Work out the finished part from the listing and answer in its coordinate system (mm). Face numbers are marked on the shaded views. A direction names the side the tool comes from. Round coordinates to 2 decimals unless told otherwise and drop trailing zeros. Loops run counter-clockwise (first coordinate to the right, second up) from the corner with the lowest first, then second, coordinate; pieces in that order, holes last. Notation, with made-up numbers: (-21, -1.5) - (30, -1.5) arc R28 cw to (30, 37.5) - close; hole circle Ø4 at (-20.5, 11.5). An arc over 180 degrees is marked (long way). Answer as CSV lines item,"result". Start each with the question number.
Q1. For the marked faces 1, 2 and 3, determine the directions among +Z, -Z, +X, -X, +Y, -Y from which every point of the face is accessible in a straight line to the end or side of a thin tool.
Q2. Section A-A on z = -5 is taken. Write down the section's boundary in (x, y), then the cut area to 3 significant figures.
Q3. Section C-C on y = 0.5 is taken. Write down the section's boundary in (x, z) (3 decimals), then the cut area to 3 significant figures.
Q4. Straight lines are drawn through the part: L1, parallel to X at y = 1.5, z = 17.78 (3 decimals); L2, parallel to Z at x = -20.32, y = -1.75; L3, parallel to X at y = 0.25, z = 4.5. For each, find the intervals that lie inside material, in ascending order. Write a range as [from, to].
Q5. Each of these flat-tipped pins is pushed along its axis until it touches: pin 1 Ø3 at (x, z) = (-17, -1) entering from -Y; pin 2 Ø1.4 at (x, z) = (-20.32, -17.78) entering from -Y; pin 3 Ø3 at (x, y) = (-2, 2) entering from -Z; pin 4 Ø3.5 at (y, z) = (-1, 18.5) entering from +X. Where does it stop, or does it pass through?
Q6. Section B-B on x = 0 is taken. Write down the section's boundary in (y, z).
Q7. The mould has two halves that part along X. Classify the marked faces 4, 5 and 6: +X half, -X half, draft (parallel to the pull), parting line (faces both ways), or undercut.
Q8. Section D-D on y = -6 is taken. Write down the section's boundary in (x, z), then the cut area to 3 significant figures.
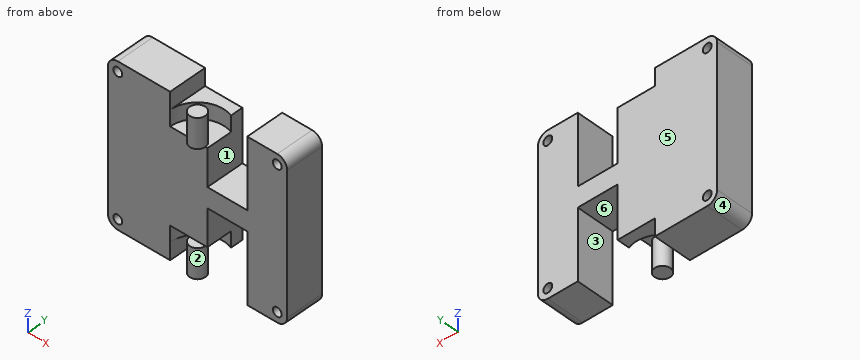
```python
from build123d import *

# Parameters (mm, degrees)
SKETCH1_W             = 45.72
SKETCH1_H             = 40.64
BODY_DEPTH            = 4.826
CORNER_FILLET_R       = 2.54
F_4_40_TAPPED_HOLE1_D = 2.2606
SKETCH4_W             = 13.97
SKETCH4_H             = 9.652
WHEEL_CUTOUT_DEPTH    = 8.382
SKETCH5_R             = 2
WHEEL_SHAFT_DEPTH     = 7.5
SKETCH9_W             = 10.16
SKETCH9_H             = 9.652
CUT_EXTRUDE2_DEPTH    = 17.78
BOSS_EXTRUDE2_DEPTH   = 4


with BuildPart() as part:
    # Sketch1 → Body (new body, symmetric)
    with BuildSketch(Plane(origin=(0, 0, 0), x_dir=(1, 0, 0), z_dir=(0, 1, 0))):
        Rectangle(SKETCH1_W, SKETCH1_H)
    extrude(amount=BODY_DEPTH, both=True)

    # Corner Fillet
    corner_fillet_edges = [part.edges().sort_by_distance(p)[0] for p in [
        (22.86, 0, 20.32),
        (-22.86, 0, 20.32),
        (-22.86, 0, -20.32),
        (22.86, 0, -20.32),
    ]]
    fillet(corner_fillet_edges, radius=CORNER_FILLET_R)

    # #4-40 Tapped Hole1 (through all)
    with Locations(Plane(origin=(0, 4.826, 0), x_dir=(1, 0, 0), z_dir=(0, 1, 0))):
        with Locations((20.32, 17.78), (-20.32, -17.78), (-20.32, 17.78), (20.32, -17.78)):
            Hole(F_4_40_TAPPED_HOLE1_D / 2)

    # Sketch4 → Wheel Cutout (cut)
    with BuildSketch(Plane(origin=(0, 0, -20.32), x_dir=(-1, 0, 0), z_dir=(0, 0, -1))):
        Rectangle(SKETCH4_W, SKETCH4_H)
    wheel_cutout = extrude(amount=-WHEEL_CUTOUT_DEPTH, mode=Mode.SUBTRACT)

    # Sketch5 → Wheel Shaft (add)
    with BuildSketch(Plane(origin=(0, 0, -11.938), x_dir=(-1, 0, 0), z_dir=(0, 0, -1))):
        with Locations((0, -4.826)):
            Circle(SKETCH5_R)
    wheel_shaft = extrude(amount=WHEEL_SHAFT_DEPTH)

    # Sketch9 → Cut-Extrude2 (cut)
    with BuildSketch(Plane(origin=(0, 0, -20.32), x_dir=(-1, 0, 0), z_dir=(0, 0, -1))):
        with Locations((-7.603288762, 0)):
            Rectangle(SKETCH9_W, SKETCH9_H)
    cut_extrude2 = extrude(amount=-CUT_EXTRUDE2_DEPTH, mode=Mode.SUBTRACT)

    # Sketch10 → Boss-Extrude2 (add)
    with BuildSketch(Plane(origin=(0, 0, -11.938), x_dir=(-1, 0, 0), z_dir=(0, 0, -1))):
        with BuildLine():
            Line((6.985, 4.826), (-2.523288762, 4.826))
            Line((-2.523288762, 4.826), (-2.523288762, 1.687312431))
            ThreePointArc((-2.523288762, 1.687312431), (3.947470899, 0.936612125), (6.985, -4.826))
            Line((6.985, -4.826), (6.985, 4.826))
        make_face()
    boss_extrude2 = extrude(amount=BOSS_EXTRUDE2_DEPTH)

    # Mirror3: Wheel Cutout, Wheel Shaft, Cut-Extrude2, Boss-Extrude2 across plane
    add(wheel_cutout.mirror(Plane.XY), mode=Mode.SUBTRACT)
    add(wheel_shaft.mirror(Plane.XY))
    add(cut_extrude2.mirror(Plane.XY), mode=Mode.SUBTRACT)
    add(boss_extrude2.mirror(Plane.XY))


solid = part.part
```
Findings:
1,face 1,"+Z, +Y, -Y"
1,face 2,"-Z"
1,face 3,"-Z, +Y, -Y"
2,outline,"(-22.86, -4.83) - (2.52, -4.83) - (2.52, 4.83) - (-22.86, 4.83) - close; (12.68, -4.83) - (22.86, -4.83) - (22.86, 4.83) - (12.68, 4.83) - close"
2,area,"343 mm^2"
3,outline,"(-22.86, -17.78) arc R2.54 ccw to (-20.32, -20.32) - (-6.985, -20.32) - (-6.985, -15.938) - (-4.519, -15.938) - (-4.519, -11.938) - (2.523, -11.938) - (2.523, -2.54) - (12.683, -2.54) - (12.683, -20.32) - (20.32, -20.32) arc R2.54 ccw to (22.86, -17.78) - (22.86, 17.78) arc R2.54 ccw to (20.32, 20.32) - (12.683, 20.32) - (12.683, 2.54) - (2.523, 2.54) - (2.523, 11.938) - (-4.519, 11.938) - (-4.519, 15.938) - (-6.985, 15.938) - (-6.985, 20.32) - (-20.32, 20.32) arc R2.54 ccw to (-22.86, 17.78) - close; hole circle Ø2.261 at (-20.32, -17.78); hole circle Ø2.261 at (-20.32, 17.78); hole circle Ø2.261 at (20.32, -17.78); hole circle Ø2.261 at (20.32, 17.78)"
3,area,"1,340 mm^2"
4,L1,"x = [-22.86, -21.45], [-19.19, -6.985], [12.683, 19.19], [21.45, 22.86]"
4,L2,"z = [-20.32, -18.91], [-16.65, 16.65], [18.91, 20.32]"
4,L3,"x = [-22.86, 2.52], [12.68, 22.86]"
5,pin 1,"stops at y = -4.83"
5,pin 2,"passes through"
5,pin 3,"stops at z = -15.94"
5,pin 4,"stops at x = 22.86"
6,outline,"(-6.83, -19.44) - (-2.83, -19.44) - (-2.83, -11.94) - (2.16, -11.94) - (2.16, -15.94) - (4.83, -15.94) - (4.83, 15.94) - (2.16, 15.94) - (2.16, 11.94) - (-2.83, 11.94) - (-2.83, 19.44) - (-6.83, 19.44) - (-6.83, 11.94) - (-4.83, 11.94) - (-4.83, -11.94) - (-6.83, -11.94) - close"
7,face 4,"-X half"
7,face 5,"draft"
7,face 6,"undercut"
8,outline,"(-1.62, -19.44) - (1.62, -19.44) - (1.62, -11.94) - (-1.62, -11.94) - close; (-1.62, 11.94) - (1.62, 11.94) - (1.62, 19.44) - (-1.62, 19.44) - close"
8,area,"48.6 mm^2"
